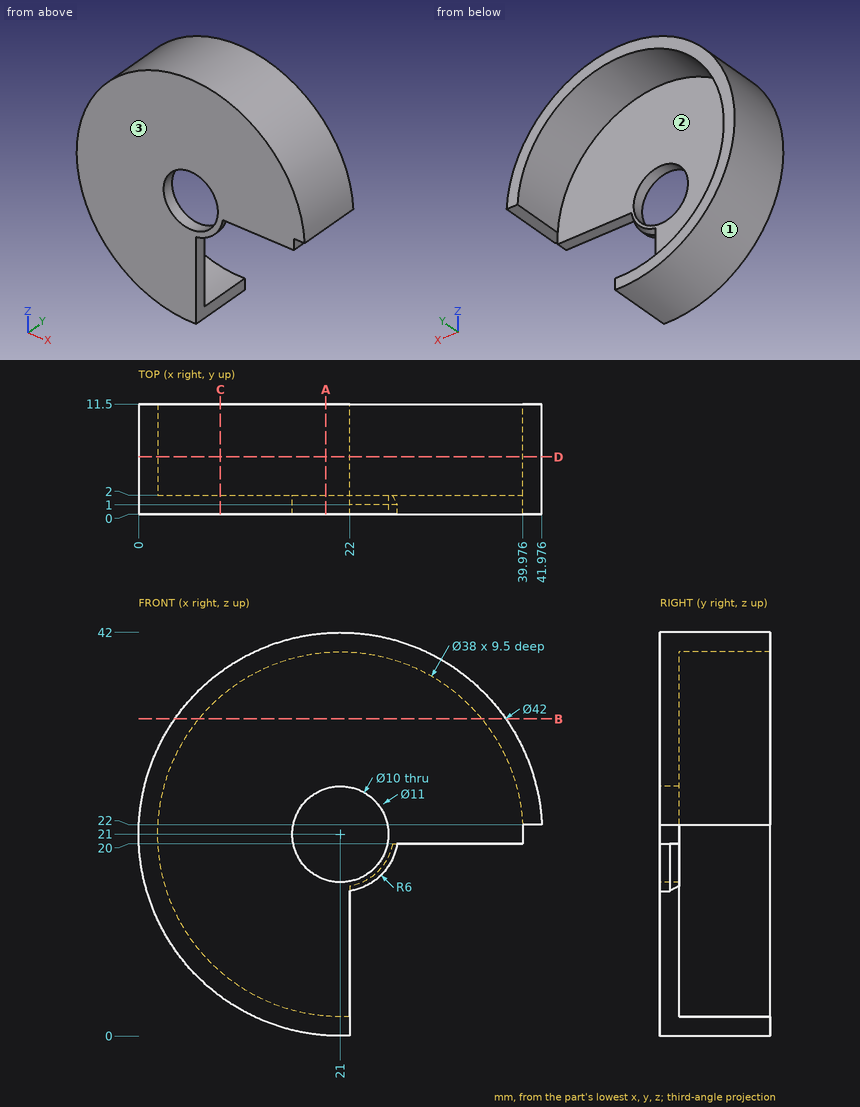
The drawing under review shows one solid part. Ordinate dimensions are in mm from its lowest x, y, z. Round coordinates to 2 decimals unless told otherwise and drop trailing zeros. Write each loop counter-clockwise with the first axis right and the second up, starting at its lowest first coordinate (ties: lowest second). Pieces come first, ordered by that corner, then holes. Notation, with made-up numbers: M 2,82 L 59,82 A25 ccw 59,121 Z; hole C -14,-8 d2. An arc over 180 degrees is marked long. One line per item, written item: value. Start each with the question number.
(1) We need section B-B (z = 33). Give the boundary of the cut face in (x, y).
(2) Insertion check: pin 1 (3.5 mm diameter, centred on y = 3.5, z = 9, fed in from +X); pin 2 (6 mm diameter, centred on x = 32, y = 9.5, fed in from -Z) (1 decimal); pin 3 (4 mm diameter, centred on x = 12, y = 4.5, fed in from +Z). Each pin has a flat end and moves straight along its axis. Give the tip position at first contact, or say it passes through.
(3) Wall thickness on line 1 (Y direction, x = 20.5, z = 13); line 2 (Z direction, x = 14, y = 6.75); line 3 (Z direction, x = 17.5, y = 10.25) (1 decimal): over which ranges is each line inside the solid? List them lowest first.
(4) We need section A-A (x = 19.5). Give the boundary of the cut face in (y, z), and give its area (3 significant figures).
(5) The part is to be moulded in two halves that separate along X. For the marked faces 1, 2 and 3, say which applies: released by +X, released by -X, zero draft, split by the parting line, or undercut.
(6) We need section D-D (y = 6). Give the boundary of the cut face in (x, z).
(7) We need section C-C (x = 8.5). Give the boundary of the cut face in (y, z) (1 decimal).
Result:
1. outline: M 3.77,0 L 38.23,0 L 38.23,11.5 L 35.73,11.5 L 35.73,2 L 6.27,2 L 6.27,11.5 L 3.77,11.5 Z
2. pin 1: x = 22
2. pin 2: z = 33.8
2. pin 3: z = 40.8
3. line 1: 0 to 2
3. line 2: 1.2 to 3.34, 38.66 to 40.8
3. line 3: 0.3 to 2.3, 39.7 to 41.7
4. outline: M 0,0.05 L 11.5,0.05 L 11.5,2.06 L 2,2.06 L 2,16.23 L 0,16.23 Z; M 0,25.77 L 2,25.77 L 2,39.94 L 11.5,39.94 L 11.5,41.95 L 0,41.95 Z
4. area: 103 mm²
5. face 1: split by the parting line
5. face 2: undercut
5. face 3: zero draft
6. outline: M 22,0.02 L 22,2.03 A19 cw long 39.97,22 L 41.98,22 A21 ccw long Z
7. outline: M 0,4.1 L 11.5,4.1 L 11.5,6.7 L 2,6.7 L 2,35.3 L 11.5,35.3 L 11.5,37.9 L 0,37.9 Z
